Work out the finished part from the listing and answer in its coordinate system (mm). A direction names the side the tool comes from. Coordinates: 2 decimals unless noted, no trailing zeros. Write each loop counter-clockwise with the first axis right and the second up, starting at its lowest first coordinate (ties: lowest second). Pieces come first, ordered by that corner, then holes. Notation, with made-up numbers: (58.25, -13.5) - (66.25, -13.5) arc R8 ccw to (66.25, -8.5) - close; hole circle Ø1 at (21.5, 3.25). An arc over 180 degrees is marked (long way). One line per item, written item: value.
```python
from build123d import *

# Parameters (mm, degrees)
MAIN_BODY_DEPTH       = 18
SKETCH14_W            = 4.2
SKETCH14_H            = 39
M8_CLEARANCE_HOLE2_D  = 8.4
M8_CLEARANCE_HOLE3_D  = 8.4
SKETCH27_R            = 7
CUT_EXTRUDE2_DEPTH    = 99.559772913
F_8_32_TAPPED_HOLE1_D = 3.4544


with BuildPart() as part:
    # Sketch1 → main body (new body)
    with BuildSketch(Plane.XY):
        with BuildLine():
            Line((0, -48.600411521), (0, -83.600411521))
            Line((0, -83.600411521), (-10, -83.600411521))
            Line((-10, -83.600411521), (-10, -48.600411521))
            add(Edge.make_bspline(
                [(-26.535230031, -29.931280748), (-20.948212629, -34.88438627), (-10, -40.904022772), (-10, -48.600411521)],
                knots=[0, 0, 0, 0, 1, 1, 1, 1], degree=3))
            ThreePointArc((-26.535230031, -29.931280748), (-39.998128482, 0.386934068), (-25.951219512, 30.43902439))
            ThreePointArc((-25.951219512, 30.43902439), (-18.607817439, 40.126684972), (-16, 52))
            Line((-16, 52), (-1, 52))
            Line((-1, 52), (-1, 29.983328701))
            ThreePointArc((-1, 29.983328701), (0, -30), (1, 29.983328701))
            Line((1, 29.983328701), (1, 52))
            Line((1, 52), (9, 52))
            ThreePointArc((9, 52), (11.695932832, 42.212959957), (19.02319236, 35.186903138))
            ThreePointArc((19.02319236, 35.186903138), (39.54457484, -6.018853774), (7.693084301, -39.253234949))
            ThreePointArc((7.693084301, -39.253234949), (2.170592409, -42.547452411), (0, -48.600411521))
        make_face()
    extrude(amount=MAIN_BODY_DEPTH)

    # Sketch14 → M8 Clearance Hole1 (revolve, cut)
    with BuildSketch(Plane(origin=(1, 43, 9), x_dir=(0, 0, 1), z_dir=(0, 1, 0))):
        with Locations((2.1, 19.5)):
            Rectangle(SKETCH14_W, SKETCH14_H)
    revolve(axis=Axis((-5.35, 43, 9), (1, 0, 0)), mode=Mode.SUBTRACT)

    # M8 Clearance Hole2 (through all)
    with Locations(Plane(origin=(1, 0, 0), x_dir=(0, 0, 1), z_dir=(1, 0, 0))):
        with Locations((9, -43)):
            Hole(M8_CLEARANCE_HOLE2_D / 2)

    # M8 Clearance Hole3 (through all)
    with Locations(Plane(origin=(0, 0, 0), x_dir=(0, 0, -1), z_dir=(1, 0, 0))):
        with Locations((-9, -53.34)):
            Hole(M8_CLEARANCE_HOLE3_D / 2)

    # Sketch27 → Cut-Extrude2 (cut, through all)
    with BuildSketch(Plane(origin=(9, 0, 0), x_dir=(0, 0, -1), z_dir=(1, 0, 0))):
        with Locations(Location((-9, 43, 0), (0, 0, 270))):
            Circle(SKETCH27_R)
    extrude(amount=CUT_EXTRUDE2_DEPTH, mode=Mode.SUBTRACT)

    # #8-32 Tapped Hole1 (through all)
    with Locations(Plane(origin=(0, 0, 0), x_dir=(0, 0, -1), z_dir=(1, 0, 0))):
        with Locations((-9, -76.2)):
            Hole(F_8_32_TAPPED_HOLE1_D / 2)


solid = part.part
```
Item 1: Section D-D, the plane y = 43 is taken. Determine the outline of the cut face in (x, z).
Evaluation:
outline: (-17.47, 0) - (-1, 0) - (-1, 4.8) - (-17.47, 4.8) - close; (-17.47, 13.2) - (-1, 13.2) - (-1, 18) - (-17.47, 18) - close; (1, 0) - (11.25, 0) - (11.25, 2) - (9, 2) - (9, 4.8) - (1, 4.8) - close; (1, 13.2) - (9, 13.2) - (9, 16) - (11.25, 16) - (11.25, 18) - (1, 18) - close
Item 2: Given pin 1 (6 mm diameter, centred on x = -26.5, z = 9, fed in from -Y); pin 2 (7 mm diameter, centred on y = 44, z = 11.5, fed in from +X); pin 3 (9 mm diameter, centred on y = -62, z = 11.5, fed in from -X), each flat-ended and moving along its own axis, determine where each tip first touches the part or whether it passes through.
Evaluation:
pin 1: stops at y = -32.4
pin 2: stops at x = 9
pin 3: stops at x = -10
Item 3: Section C-C, the plane x = -3 is taken. Determine the outline of the cut face in (y, z), then the cut area to 3 significant figures.
Evaluation:
outline: (-83.6, 0) - (-29.85, 0) - (-29.85, 18) - (-83.6, 18) - close; (29.85, 0) - (52, 0) - (52, 18) - (29.85, 18) - close; hole circle Ø3.45 at (-76.2, 9); hole circle Ø8.4 at (-53.34, 9); hole circle Ø8.4 at (43, 9)
area: 1,250 mm2
Item 4: Section B-B, the plane x = 13 is taken. Determine the outline of the cut face in (y, z), then the cut area to 3 significant figures.
Evaluation:
outline: (-37.83, 0) - (-27.04, 0) - (-27.04, 18) - (-37.83, 18) - close; (27.04, 0) - (40.3, 0) - (40.3, 2.54) arc R7 cw to (40.3, 15.46) - (40.3, 18) - (27.04, 18) - close
area: 393 mm2
Item 5: Section A-A, the plane y = -76.2 is taken. Determine the outline of the cut face in (x, z), then the cut area to 3 significant figures.
Evaluation:
outline: (-10, 0) - (0, 0) - (0, 7.27) - (-10, 7.27) - close; (-10, 10.73) - (0, 10.73) - (0, 18) - (-10, 18) - close
area: 145 mm2
Item 6: Which of the six approach directions +Z, -Z, +X, -X, +Y, -Y give full straight-line access (tool end or side, diameter ignored) to faces 1 (the face through (-10, -66, 9)), 2 (the face through (0, -66, 9)), 3 (the face through (-1, 39, 11)), 4 (the face through (9, 43, 14))?
Evaluation:
face 1: +Z, -Z, -X, -Y
face 2: +Z, -Z, +X, -Y
face 3: +Z, -Z, +Y
face 4: +X
Item 7: Determine the mould class of faces 5 (the face through (-19.95, 37.57, 8.87)), 6 (the face through (-1.31, -29.97, 8.87)), 7 (the face through (-10.261, 38.836, 9.547)) for opening direction X: +X half, -X half, draft (parallel to the pull), parting line (faces both ways), or undercut.
Evaluation:
face 5: -X half
face 6: undercut
face 7: draft
Item 8: Consider probe 1 along Y at (x, z) = (8, 12.5); probe 2 along Y at (x, z) = (-4, 9); probe 3 along X at (y, z) = (-1.5, 17). Determine where each line is inside the solid, lowest interval first.
Evaluation:
probe 1: y = -39.19 to -28.91, 28.91 to 40.68, 45.32 to 52
probe 2: y = -83.6 to -77.93, -74.47 to -57.54, -49.14 to -29.73, 29.73 to 38.8, 47.2 to 52
probe 3: x = -39.97 to -29.96, 29.96 to 39.97
